```python
from build123d import *

# Parameters (mm, degrees)
BOSS_EXTRUDE1_DEPTH = 60
SKETCH2_R           = 8
SKETCH2_R_2         = 6
CUT_EXTRUDE1_DEPTH  = 1899
SKETCH3_R           = 8
SKETCH3_R_2         = 6
CUT_EXTRUDE2_DEPTH  = 1899


with BuildPart() as part:
    # Sketch1 → Boss-Extrude1 (new body)
    with BuildSketch(Plane.XY):
        Polygon((265.096679919, 640), (-265.096679919, 640), (-640, 265.096679919), (-640, -265.096679919), (-265.096679919, -640), (265.096679919, -640), (640, -265.096679919), (640, 265.096679919), align=None)
        Polygon((600, -248.528137424), (600, 248.528137424), (248.528137424, 600), (-248.528137424, 600), (-600, 248.528137424), (-600, -248.528137424), (-248.528137424, -600), (248.528137424, -600), align=None, mode=Mode.SUBTRACT)
    extrude(amount=BOSS_EXTRUDE1_DEPTH)

    # Sketch2 → Cut-Extrude1 (cut)
    with BuildSketch(Plane(origin=(640, 0, 0), x_dir=(0, 0, -1), z_dir=(1, 0, 0))):
        with Locations((-30, 0)):
            Circle(SKETCH2_R)
        with Locations((-30, 45)):
            Circle(SKETCH2_R_2)
        with Locations((-30, -45)):
            Circle(SKETCH2_R_2)
    extrude(amount=-CUT_EXTRUDE1_DEPTH, mode=Mode.SUBTRACT)

    # Sketch3 → Cut-Extrude2 (cut)
    with BuildSketch(Plane.XZ.offset(640)):
        with Locations(Location((0, 30, 0), (0, 0, 270))):
            Circle(SKETCH3_R)
        with Locations(Location((-45, 30, 0), (0, 0, 270))):
            Circle(SKETCH3_R_2)
        with Locations(Location((45, 30, 0), (0, 0, 270))):
            Circle(SKETCH3_R_2)
    extrude(amount=-CUT_EXTRUDE2_DEPTH, mode=Mode.SUBTRACT)


solid = part.part
```
Geometry: final body of the model. Coordinates: model frame, mm. A direction names the side the tool comes from. Round coordinates to 2 decimals unless told otherwise and drop trailing zeros. Order: outer loops, then holes, each group sorted by start corner. A loop starts at its lowest first (then second) coordinate and runs counter-clockwise, first axis right, second up. Notation, with made-up numbers: (71, 63.25) -> (82, 63.25) arc R9 cw to (82, 75.25) -> close; hole circle Ø3 at (66.5, -21). An arc over 180 degrees is marked (long way). Use one line per item in the form item = value. Start each with the question number.
1. Reachability of faces 4 (the face through (426.724, 421.804, 29.58)), 5 (the face through (-430, -424, 60)) from +Z, -Z, +X, -X, +Y, -Y: full face, straight path, thin tool, end or side. Return the list, or none.
2. Draft query along Y for faces 1 (the face through (449.924, -455.173, 29.58)), 2 (the face through (-426.724, -421.804, 29.58)), 3 (the face through (455.173, 449.924, 29.58)). Return one class per face: pulls with the +Y half, pulls with the -Y half, needs draft (parallel to the pull), parting line crosses it, or undercut.
3. Cut plane A-A (x = -216). Return the cut outline in (y, z).
4. Line query: probe 1 along X at (y, z) = (43, 46.5); probe 2 along X at (y, z) = (-613.5, 30). Output: solid intervals per line, ascending.
5. Pin query (flat end, axial travel): pin 1 Ø3 at (y, z) = (-431, 15) entering from +X; pin 2 Ø9.5 at (y, z) = (45, 30) entering from -X; pin 3 Ø8 at (y, z) = (484, 28.5) entering from -X; pin 4 Ø10 at (x, z) = (-314, 52.5) entering from +Y. Return the tip coordinate at first contact, or that it passes through.
Solution:
q1.face_4 = +Z, -Z
q1.face_5 = +Z, +X, -X, +Y, -Y
q2.face_1 = pulls with the -Y half
q2.face_2 = undercut
q2.face_3 = pulls with the +Y half
q3.outline = (-640, 0) -> (-600, 0) -> (-600, 60) -> (-640, 60) -> close; (600, 0) -> (640, 0) -> (640, 60) -> (600, 60) -> close
q4.probe_1 = -640 to -600, 600 to 640
q4.probe_2 = -291.6 to -51, -39 to -8, 8 to 39, 51 to 291.6
q5.pin_1 = 475.6
q5.pin_2 = through
q5.pin_3 = -425.1
q5.pin_4 = 596.1
